from build123d import *

# Parameters (mm, degrees)
SKETCH2_W           = 25
SKETCH2_H           = 37.1
BOSS_EXTRUDE2_DEPTH = 2
SKETCH2_9_W         = 5
SKETCH2_9_H         = 5
SKETCH2_9_R         = 0.85
BOSS_EXTRUDE4_DEPTH = 6
SKETCH2_10_W        = 25
SKETCH2_10_H        = 37.1
SKETCH2_10_W_2      = 23
SKETCH2_10_H_2      = 35.1
BOSS_EXTRUDE5_DEPTH = 7
SNAP_START          = 1
SNAP_HOOK1_DEPTH    = 1
SNAP_START_2        = 1.525191878
SNAP_HOOK1_2_DEPTH  = 3.157223338
SNAP_START_3        = -1
SNAP_HOOK1_3_DEPTH  = 2
SNAP_HOOK1_4_DEPTH  = 1
LPATTERN1_START     = 1
LPATTERN1_DEPTH     = 1
LPATTERN1_START_2   = 31.525191878
LPATTERN1_2_DEPTH   = 3.157223338
LPATTERN1_START_3   = -1
LPATTERN1_3_DEPTH   = 2
LPATTERN1_4_DEPTH   = 1
SKETCH2_11_R        = 0.85
BOSS_EXTRUDE7_DEPTH = 9
SKETCH9_W           = 12
SKETCH9_H           = 4.478730726
CUT_EXTRUDE2_DEPTH  = 2


with BuildPart() as part:
    # Sketch2 → Boss-Extrude2 (new body)
    with BuildSketch(Plane(origin=(0, 0, 0), x_dir=(1, 0, 0), z_dir=(0, 1, 0))):
        with Locations((12.5, -18.55)):
            Rectangle(SKETCH2_W, SKETCH2_H)
    extrude(amount=-BOSS_EXTRUDE2_DEPTH)

    # Sketch2<9> → Boss-Extrude4 (add)
    # profile 1 of 3: a face of its own
    with BuildSketch(Plane(origin=(0, 0, 0), x_dir=(1, 0, 0), z_dir=(0, 1, 0))):
        with Locations((5, -5)):
            Rectangle(SKETCH2_9_W, SKETCH2_9_H)
        with Locations(Location((5, -5, 0), (0, 0, 270))):
            Circle(SKETCH2_9_R, mode=Mode.SUBTRACT)
    # profile 2 of 3: a face of its own
    with BuildSketch(Plane(origin=(0, 0, 0), x_dir=(1, 0, 0), z_dir=(0, 1, 0))):
        with Locations((20, -32.1)):
            Rectangle(SKETCH2_9_W, SKETCH2_9_H)
        with Locations(Location((20, -32.1, 0), (0, 0, 270))):
            Circle(SKETCH2_9_R, mode=Mode.SUBTRACT)
    # profile 3 of 3: a face of its own
    with BuildSketch(Plane(origin=(0, 0, 0), x_dir=(1, 0, 0), z_dir=(0, 1, 0))):
        with Locations((20, -5)):
            Rectangle(SKETCH2_9_W, SKETCH2_9_H)
        with Locations(Location((20, -5, 0), (0, 0, 270))):
            Circle(SKETCH2_9_R, mode=Mode.SUBTRACT)
    extrude(amount=BOSS_EXTRUDE4_DEPTH)

    # Sketch2<10> → Boss-Extrude5 (add)
    with BuildSketch(Plane(origin=(0, 0, 0), x_dir=(1, 0, 0), z_dir=(0, 1, 0))):
        with Locations((12.5, -18.55)):
            Rectangle(SKETCH2_10_W, SKETCH2_10_H)
        with Locations((12.5, -18.55)):
            Rectangle(SKETCH2_10_W_2, SKETCH2_10_H_2, mode=Mode.SUBTRACT)
    extrude(amount=BOSS_EXTRUDE5_DEPTH)



with BuildPart() as body_2:
    # Snap Hook1: read off the stored shape, not the designer's step
    # Snap Hook1 outline → Snap Hook1 (new body)
    with BuildSketch(Plane.YZ.offset(SNAP_START)):
        Polygon((8, 4.682415216), (8, 1.525191878), (9.5, 1.603803547), (9.5, 4.603803547), align=None)
    snap_hook1 = extrude(amount=SNAP_HOOK1_DEPTH)

    # Snap Hook1 2 outline → Snap Hook1 2 (add)
    with BuildSketch(Plane.XY.offset(SNAP_START_2)):
        Polygon((1, 8), (1, 9.5), (0, 8), align=None)
    snap_hook1_2 = extrude(amount=SNAP_HOOK1_2_DEPTH)

    # Snap Hook1 3 outline → Snap Hook1 3 (cut)
    with BuildSketch(Plane.YZ.offset(SNAP_START_3)):
        Polygon((9.5, 1.603803547), (8, 1.525191878), (11, 1.525191878), (11, 1.682415216), align=None)
        Polygon((11, 4.682415216), (8, 4.682415216), (9.5, 4.603803547), (11, 4.525191878), align=None)
    snap_hook1_3 = extrude(amount=SNAP_HOOK1_3_DEPTH, mode=Mode.SUBTRACT)


with BuildPart() as part_1:
    add(part.part)

    add(body_2.part)  # Snap Hook1 4 merges body 2
    # Snap Hook1 4 outline → Snap Hook1 4 (add)
    with BuildSketch(Plane.YZ.offset(SNAP_START)):
        Polygon((-1, 1.053521865), (0, 1.105929644), (8, 1.525191878), (8, 4.682415216), (0, 5.10167745), (-1, 5.154085229), align=None)
    snap_hook1_4 = extrude(amount=SNAP_HOOK1_4_DEPTH)



with BuildPart() as body_2_2:
    # LPattern1: read off the stored shape, not the designer's step
    # LPattern1 outline → LPattern1 (new body)
    with BuildSketch(Plane.YZ.offset(LPATTERN1_START)):
        Polygon((8, 31.525191878), (9.5, 31.603803547), (9.5, 34.603803547), (8, 34.682415216), align=None)
    lpattern1 = extrude(amount=LPATTERN1_DEPTH)

    # LPattern1 2 outline → LPattern1 2 (add)
    with BuildSketch(Plane.XY.offset(LPATTERN1_START_2)):
        Polygon((1, 8), (1, 9.5), (0, 8), align=None)
    lpattern1_2 = extrude(amount=LPATTERN1_2_DEPTH)

    # LPattern1 3 outline → LPattern1 3 (cut)
    with BuildSketch(Plane.YZ.offset(LPATTERN1_START_3)):
        Polygon((9.5, 31.603803547), (8, 31.525191878), (11, 31.525191878), (11, 31.682415216), align=None)
        Polygon((11, 34.682415216), (8, 34.682415216), (9.5, 34.603803547), (11, 34.525191878), align=None)
    lpattern1_3 = extrude(amount=LPATTERN1_3_DEPTH, mode=Mode.SUBTRACT)


with BuildPart() as part_2:
    add(part_1.part)

    add(body_2_2.part)  # LPattern1 4 merges body 2 2
    # LPattern1 4 outline → LPattern1 4 (add)
    with BuildSketch(Plane.YZ.offset(LPATTERN1_START)):
        Polygon((-1, 31.053521865), (0, 31.105929644), (8, 31.525191878), (8, 34.682415216), (0, 35.10167745), (-1, 35.154085229), align=None)
    lpattern1_4 = extrude(amount=LPATTERN1_4_DEPTH)

    # Mirror1: Snap Hook1, Snap Hook1 2, Snap Hook1 3, Snap Hook1 4, LPattern1, LPattern1 2, LPattern1 3, LPattern1 4 across plane
    add(snap_hook1.mirror(Plane.ZY.offset(-12.5)))
    add(snap_hook1_2.mirror(Plane.ZY.offset(-12.5)))
    add(snap_hook1_3.mirror(Plane.ZY.offset(-12.5)), mode=Mode.SUBTRACT)
    add(snap_hook1_4.mirror(Plane.ZY.offset(-12.5)))
    add(lpattern1.mirror(Plane.ZY.offset(-12.5)))
    add(lpattern1_2.mirror(Plane.ZY.offset(-12.5)))
    add(lpattern1_3.mirror(Plane.ZY.offset(-12.5)), mode=Mode.SUBTRACT)
    add(lpattern1_4.mirror(Plane.ZY.offset(-12.5)))

    # Sketch2<11> → Boss-Extrude7 (add)
    with BuildSketch(Plane(origin=(0, 0, 0), x_dir=(1, 0, 0), z_dir=(0, 1, 0))):
        with Locations(Location((20, -32.1, 0), (0, 0, 270))):
            Circle(SKETCH2_11_R)
        with Locations(Location((5, -5, 0), (0, 0, 270))):
            Circle(SKETCH2_11_R)
        with Locations(Location((20, -5, 0), (0, 0, 270))):
            Circle(SKETCH2_11_R)
    extrude(amount=BOSS_EXTRUDE7_DEPTH)

    # Sketch9 → Cut-Extrude2 (cut)
    with BuildSketch(Plane.XY.offset(37.1)):
        with Locations((12.5, 2.5)):
            Rectangle(SKETCH9_W, SKETCH9_H)
    extrude(amount=-CUT_EXTRUDE2_DEPTH, mode=Mode.SUBTRACT)


solid = part_2.part
Geometry check sheet. Reference: the model listing, model coordinates, mm. A direction names the side the tool comes from. Round coordinates to 2 decimals unless told otherwise and drop trailing zeros. Write each loop counter-clockwise with the first axis right and the second up, starting at its lowest first coordinate (ties: lowest second). Pieces come first, ordered by that corner, then holes. Notation, with made-up numbers: (25, 12.5) -> (74, 12.5) arc R21 cw to (74, 51.5) -> close; hole circle Ø9 at (-32, 61.25). An arc over 180 degrees is marked (long way). One line per item, written item: value. Start each with the question number.
(1) Scan lines: line 1 (Z direction, x = 5, y = 4.75); line 2 (X direction, y = 3, z = 32.5); line 3 (X direction, y = 5.75, z = 13). Record each from-to range of solid material in increasing order. Write a range as [from, to].
(2) Cross-section at D-D, the plane y = 3.75. Give the number of separate pieces and of enclosed holes in the cut face, and give its area (3 significant figures).
(3) Draft check along Z on faces 1 (the flat face through (12, 5, 36.1)), 2 (the flat face through (12, 5, 37.1)), 3 (the flat face through (20, 3, 29.6)), 4 (the flat face through (24.493, 8.76, 3.082)). Enter one of: +Z half, -Z half, draft (parallel to the pull), parting line (faces both ways), or undercut.
(4) Access from +Z, -Z, +X, -X, +Y, -Y to the whole of each face (thin tool, end or side, straight path). Record for faces 5 (the flat face through (24.5, 8, 33.1)), 6 (the flat face through (20, 9, 5)), 7 (the flat face through (24.493, 8.76, 33.082)), 8 (the flat face through (18.5, 2.5, 36.6)), 9 (the flat face through (24, 3.5, 35.6)).
(5) Cross-section at A-A, the plane x = 10.5. Record the cut outline in (y, z).
(6) Cross-section at C-C, the plane z = 25. Record the cut outline in (x, y), and give its area (3 significant figures).
(7) Cross-section at B-B, the plane x = 5. Record the cut outline in (y, z), and give its area (3 significant figures).
(8) Go/stop test with a flat-tipped pin: pin 1 Ø2 at (x, z) = (5, 28) entering from +Y. Record where the tip stops, or that it passes through.
Answer:
1. line 1: [0, 1], [2.5, 7.5], [36.1, 37.1]
1. line 2: [0, 2], [17.5, 22.5], [23, 25]
1. line 3: [0, 1], [24, 25]
2. separate pieces: 4
2. enclosed holes: 0
2. area: 198 mm²
3. face 1: undercut
3. face 2: +Z half
3. face 3: undercut
3. face 4: draft
4. face 5: +Z, -Z, +X
4. face 6: +Z, -Z, +Y
4. face 7: +Z, -Z, +X, +Y
4. face 8: +Z
4. face 9: +Y
5. outline: (-2, 0) -> (7, 0) -> (7, 1) -> (0, 1) -> (0, 36.1) -> (0.26, 36.1) -> (0.26, 37.1) -> (-2, 37.1) -> close; (4.74, 36.1) -> (7, 36.1) -> (7, 37.1) -> (4.74, 37.1) -> close
6. outline: (0, -2) -> (25, -2) -> (25, 7) -> (24, 7) -> (24, 0) -> (1, 0) -> (1, 7) -> (0, 7) -> close
6. area: 64.0 mm²
7. outline: (-2, 0) -> (7, 0) -> (7, 1) -> (0, 1) -> (0, 2.5) -> (6, 2.5) -> (6, 4.15) -> (9, 4.15) -> (9, 5.85) -> (6, 5.85) -> (6, 7.5) -> (0, 7.5) -> (0, 36.1) -> (7, 36.1) -> (7, 37.1) -> (-2, 37.1) -> close
7. area: 123 mm²
8. pin 1: y = 0
